from build123d import *

# Parameters (mm, degrees)
SKETCH1_W                   = 50
SKETCH1_H                   = 41
BOSS_EXTRUDE1_DEPTH         = 30
SKETCH8_R                   = 14
SKETCH8_W                   = 24
SKETCH8_H                   = 4
CUT_EXTRUDE1_DEPTH          = 45.10498838
TAP_DRILL_FOR_M4_TAP1_D     = 3.3
TAP_DRILL_FOR_M5_TAP2_D     = 4.2
TAP_DRILL_FOR_M5_TAP2_DEPTH = 15
TAP_DRILL_FOR_M5_TAP2_TIP   = 1.2618073
CHAMFER1_SIZE               = 2
CHAMFER2_SIZE               = 10


with BuildPart() as part:
    # Sketch1 → Boss-Extrude1 (new body)
    with BuildSketch(Plane.XY):
        Rectangle(SKETCH1_W, SKETCH1_H)
    extrude(amount=BOSS_EXTRUDE1_DEPTH)

    # Sketch8 → Cut-Extrude1 (cut, through all)
    with BuildSketch(Plane.XY.offset(30)):
        with Locations((0, -2.5)):
            Circle(SKETCH8_R)
        with Locations((0, 20.5)):
            Rectangle(SKETCH8_W, SKETCH8_H)
    extrude(amount=-CUT_EXTRUDE1_DEPTH, mode=Mode.SUBTRACT)

    # Tap Drill for M4 Tap1 (through all)
    with Locations(Plane.XY.offset(30)):
        with Locations((19, -2.5), (-19, -2.5)):
            Hole(TAP_DRILL_FOR_M4_TAP1_D / 2)

    # Tap Drill for M5 Tap2
    with Locations(Plane(origin=(0, 20.5, 0), x_dir=(1, 0, 0), z_dir=(0, 1, 0))):
        with Locations((-18, -25), (-18, -5), (18, -5), (18, -25)):
            Hole(TAP_DRILL_FOR_M5_TAP2_D / 2, depth=TAP_DRILL_FOR_M5_TAP2_DEPTH)
            with Locations((0, 0, -(TAP_DRILL_FOR_M5_TAP2_DEPTH + TAP_DRILL_FOR_M5_TAP2_TIP / 2))):  # 118° drill point
                Cone(0, TAP_DRILL_FOR_M5_TAP2_D / 2, TAP_DRILL_FOR_M5_TAP2_TIP, mode=Mode.SUBTRACT)

    # Chamfer1
    chamfer1_edges = [part.edges().sort_by_distance(p)[0] for p in [
        (12, 18.5, 15),
        (-12, 18.5, 15),
    ]]
    chamfer(chamfer1_edges, length=CHAMFER1_SIZE - 0.0001)  # a hair under: the kernel refuses the full size

    # Chamfer2
    chamfer2_edges = [part.edges().sort_by_distance(p)[0] for p in [
        (25, -20.5, 15),
        (-25, -20.5, 15),
    ]]
    chamfer(chamfer2_edges, length=CHAMFER2_SIZE)


solid = part.part
Can you work these out from the model? Positions are in its coordinate system, mm. A direction names the side the tool comes from. Give positions to 0.01 mm unless a question says otherwise; leave off trailing zeros. Order: outer loops, then holes, each group sorted by start corner. A loop starts at its lowest first (then second) coordinate and runs counter-clockwise, first axis right, second up. Notation, with made-up numbers: M -24.75,-23.5 L -16.75,-23.5 A26 cw -16.75,2.5 Z; hole C -37.5,74 d2. An arc over 180 degrees is marked long. Use one line per item in the form item = value. Start each with the question number.
Item 1: Will these pins go through, and if not, where does the flat tip stop? pin 1 Ø3 at (x, y) = (-19, -2.5) entering from -Z; pin 2 Ø6 at (x, z) = (-1.5, 20) entering from +Y; pin 3 Ø5 at (x, z) = (18, 25) entering from -Y; pin 4 Ø3.5 at (x, z) = (18, 5) entering from +Y.
Item 2: If we section it at D-D (y = 13.5): Write out the boundary of the cut face in (x, z), then the cut area to 3 significant figures.
Item 3: If we section it at B-B (z = 19.5): State how many separate pieces and enclosed holes the cut face has, then the cut area to 3 significant figures.
Item 4: If we section it at A-A (y = 8.5): Write out the boundary of the cut face in (x, z), then the cut area to 3 significant figures.
Item 5: For faces 1 (the cylindrical face through (15.997, 12.895, 24.369)), 2 (the cylindrical face through (20.31, -3.5, 14.79)), 3 (the flat face through (11, 19.5, 15.2)), which set-ups out of +Z, -Z, +X, -X, +Y, -Y let a thin tool reach every point of the face, with its end or its side?
Item 6: If we section it at C-C (x = 3.5): Write out the boundary of the cut face in (y, z).
Item 7: If I drill on line 1 along Z through (x, y) = (18, 12); line 2 along Y through (x, z) = (0, 12); line 3 along X through (y, z) = (16, 25), over which ranges is the centre line in solid material (lowest first)?
Item 8: We'd pull the mould along X, two halves only. Please class faces 4 (the flat face through (25, 5, 15)), 5 (the flat face through (0, 14, 0)), 6 (the flat face through (0, 18.5, 15)): +X half, -X half, draft (parallel to the pull), parting line (faces both ways), or undercut.
Outcome:
q1.pin_1 = through
q1.pin_2 = 18.5
q1.pin_3 = -20
q1.pin_4 = 5.29
q2.outline = M -25,0 L 25,0 L 25,30 L -25,30 Z; hole C -18,5 d4.2; hole C -18,25 d4.2; hole C 18,5 d4.2; hole C 18,25 d4.2
q2.area = 1,440 mm2
q3.separate_pieces = 1
q3.enclosed_holes = 3
q3.area = 1,270 mm2
q4.outline = M -25,0 L -8.66,0 L -8.66,30 L -25,30 Z; M 8.66,0 L 25,0 L 25,30 L 8.66,30 Z; hole C -18,5 d4.2; hole C -18,25 d4.2; hole C 18,5 d4.2; hole C 18,25 d4.2
q4.area = 925 mm2
q5.face_1 = +Y
q5.face_2 = +Z, -Z
q5.face_3 = +Z, -Z, +Y
q6.outline = M -20.5,0 L -16.06,0 L -16.06,30 L -20.5,30 Z; M 11.06,0 L 18.5,0 L 18.5,30 L 11.06,30 Z
q7.line_1 = 0 to 2.9, 7.1 to 22.9, 27.1 to 30
q7.line_2 = -20.5 to -16.5, 11.5 to 18.5
q7.line_3 = -25 to -20.1, -15.9 to 15.9, 20.1 to 25
q8.face_4 = +X half
q8.face_5 = draft
q8.face_6 = undercut
